Verification items for the finished model (mm, model axes). Face numbers are marked on the shaded views. Coordinates: 2 decimals unless noted, no trailing zeros. Write each loop counter-clockwise with the first axis right and the second up, starting at its lowest first coordinate (ties: lowest second). Pieces come first, ordered by that corner, then holes. Notation, with made-up numbers: (37.25, -5.5) - (50.25, -5.5) arc R9 ccw to (50.25, 8.5) - close; hole circle Ø4 at (-20.5, 58). An arc over 180 degrees is marked (long way). Use one line per item in the form item = value. Start each with the question number.
(1) Material ranges on line 1 (Z direction, x = 13.25, y = -5.5); line 2 (X direction, y = -7, z = 1.65); line 3 (X direction, y = -2, z = 0.5) (3 decimals), recorded low to high. Write a range as [from, to].
(2) Sectioned sample at C-C (x = 7.75). Record the cut outline in (y, z) (3 decimals), and give its area (3 significant figures).
(3) Sectioned sample at D-D (z = 3.75). Record the cut outline in (x, y), and give its area (3 significant figures).
(4) Gauge pin test, flat ends, axial feed: pin 1 Ø2.5 at (x, z) = (0, 2) entering from -Y; pin 2 Ø1.5 at (y, z) = (-5, 2.5) entering from -X; pin 3 Ø0.7 at (x, y) = (-0.5, -7) entering from +Z; pin 4 Ø0.6 at (x, y) = (3, -2) entering from -Z. Record the tip position at first contact, or that the pin passes through.
(5) Mould release check, pull along X, two halves, no side actions. Record for the marked faces 1, 2 and 3: released by +X, released by -X, zero draft, split by the parting line, or undercut.
(6) Sectioned sample at A-A (x = 0.5). Record the cut outline in (y, z).
(7) Sectioned sample at B-B (y = -3.25). Record the cut outline in (x, z) (3 decimals).
from build123d import *
from OCP.BRepFilletAPI import BRepFilletAPI_MakeChamfer

# Parameters (mm, degrees)
SKETCH_1_W             = 9.65
SKETCH_1_H             = 10.67
EXTRUDE_1_DEPTH        = 4.67
SKETCH_2_W             = 1.4
SKETCH_2_H             = 10.67
EXTRUDE_2_DEPTH        = 1.65
CHAMFER_1_SIZE         = 0.9
CHAMFER_1_SIZE2        = 2.472729678
CHAMFER_2_SIZE         = 3.22
CHAMFER_2_SIZE2        = 0.509997898
CHAMFER_3_SIZE         = 2.5
CHAMFER_3_SIZE2        = 0.395961101
FILLET_1_R             = 0.1
EXTRUDE_2_2_DEPTH      = 0.45
PATTERN_LINEAR_1_COUNT = 5
PATTERN_LINEAR_1_PITCH = 1.7


with BuildPart() as part:
    # Эскиз1 → Бобышка-Вытянуть1 (new body)
    with BuildSketch(Plane.XY):
        Rectangle(SKETCH_1_W, SKETCH_1_H)
    extrude(amount=EXTRUDE_1_DEPTH)

    # Эскиз2 → Extrude 2 (add)
    with BuildSketch(Plane(origin=(4.825, 0, 0), x_dir=(0, 0, -1), z_dir=(1, 0, 0))):
        with Locations((-0.7, 0)):
            Rectangle(SKETCH_2_W, SKETCH_2_H)
    extrude(amount=EXTRUDE_2_DEPTH)

    # Фаска1: one chamfer whose edges measure the first distance from different faces: ONE call of the kernel's chamfer builder (chamfer() names one face for all edges)
    chamfer_1_edges_1 = [part.edges().sort_by_distance(p)[0] for p in [
        (6.475, 5.335, 0.7),
    ]]
    chamfer_1_side_1 = [part.faces().sort_by_distance(p)[0] for p in [
        (0.275490496, 5.335, 2.255278414),
    ]]
    chamfer_1_edges_2 = [part.edges().sort_by_distance(p)[0] for p in [
        (6.475, -5.335, 0.7),
    ]]
    chamfer_1_side_2 = [part.faces().sort_by_distance(p)[0] for p in [
        (0.275490496, -5.335, 2.255278414),
    ]]
    chamfer_1 = BRepFilletAPI_MakeChamfer(part.part.solid().wrapped)
    for e in chamfer_1_edges_1:
        chamfer_1.Add(CHAMFER_1_SIZE, CHAMFER_1_SIZE2, e.wrapped, chamfer_1_side_1[0].wrapped)  # the first distance lies on this face
    for e in chamfer_1_edges_2:
        chamfer_1.Add(CHAMFER_1_SIZE, CHAMFER_1_SIZE2, e.wrapped, chamfer_1_side_2[0].wrapped)  # the first distance lies on this face
    add(Compound.cast(chamfer_1.Shape()), mode=Mode.REPLACE)

    # Фаска2: one chamfer whose edges measure the first distance from different faces: ONE call of the kernel's chamfer builder (chamfer() names one face for all edges)
    chamfer_2_edges_1 = [part.edges().sort_by_distance(p)[0] for p in [
        (0, -5.335, 4.67),
    ]]
    chamfer_2_side_1 = [part.faces().sort_by_distance(p)[0] for p in [
        (0.118398369, -5.335, 2.29777282),
    ]]
    chamfer_2_edges_2 = [part.edges().sort_by_distance(p)[0] for p in [
        (0, 5.335, 4.67),
    ]]
    chamfer_2_side_2 = [part.faces().sort_by_distance(p)[0] for p in [
        (0.118398369, 5.335, 2.29777282),
    ]]
    chamfer_2_edges_3 = [part.edges().sort_by_distance(p)[0] for p in [
        (4.825, 0, 4.67),
    ]]
    chamfer_2_side_3 = [part.faces().sort_by_distance(p)[0] for p in [
        (4.825, 0, 3.035),
    ]]
    chamfer_2 = BRepFilletAPI_MakeChamfer(part.part.solid().wrapped)
    for e in chamfer_2_edges_1:
        chamfer_2.Add(CHAMFER_2_SIZE, CHAMFER_2_SIZE2, e.wrapped, chamfer_2_side_1[0].wrapped)  # the first distance lies on this face
    for e in chamfer_2_edges_2:
        chamfer_2.Add(CHAMFER_2_SIZE, CHAMFER_2_SIZE2, e.wrapped, chamfer_2_side_2[0].wrapped)  # the first distance lies on this face
    for e in chamfer_2_edges_3:
        chamfer_2.Add(CHAMFER_2_SIZE, CHAMFER_2_SIZE2, e.wrapped, chamfer_2_side_3[0].wrapped)  # the first distance lies on this face
    add(Compound.cast(chamfer_2.Shape()), mode=Mode.REPLACE)

    # Фаска3
    chamfer_3_edges = [part.edges().sort_by_distance(p)[0] for p in [
        (-4.825, 0, 0),
    ]]
    chamfer_3_side = [part.faces().sort_by_distance(p)[0] for p in [
        (-4.825, 0, 2.292002655),
    ]]
    chamfer(chamfer_3_edges, length=CHAMFER_3_SIZE, length2=CHAMFER_3_SIZE2, reference=chamfer_3_side[0])

    # Скругление1
    fillet_1_edges = [part.edges().sort_by_distance(p)[0] for p in [
        (-4.825, 0, 4.67),
        (4.315002102, 0, 4.67),
        (-0.254998949, 4.825002102, 4.67),
        (-0.254998949, -4.825002102, 4.67),
    ]]
    fillet(fillet_1_edges, radius=FILLET_1_R)

    # Эскиз6 → Extrude 2 2 (add, symmetric)
    with BuildSketch(Plane(origin=(0, 3.4, 0), x_dir=(-1, 0, 0), z_dir=(0, 1, 0))):
        with BuildLine():
            Line((4.825, 2.47), (5.572169718, 2.47))
            ThreePointArc((5.572169718, 2.47), (6.020070605, 2.307944974), (6.26058695, 1.896813701))
            Line((6.26058695, 1.896813701), (6.50441305, 0.573186299))
            ThreePointArc((6.50441305, 0.573186299), (6.744929395, 0.162055026), (7.192830282, 0))
            Line((7.192830282, 0), (9.4, 0))
            Line((9.4, 0), (9.4, 0.58))
            Line((9.4, 0.58), (7.192830282, 0.58))
            ThreePointArc((7.192830282, 0.58), (7.116047273, 0.607780862), (7.074815899, 0.678260508))
            Line((7.074815899, 0.678260508), (6.830989799, 2.00188791))
            ThreePointArc((6.830989799, 2.00188791), (6.391188483, 2.75367081), (5.572169718, 3.05))
            Line((5.572169718, 3.05), (4.825, 3.05))
            Line((4.825, 3.05), (4.825, 2.47))
        make_face()
    extrude_2_2 = extrude(amount=EXTRUDE_2_2_DEPTH, both=True)

    # Линейный массив1: Extrude 2 2 ×5
    with Locations(*[(0, -i * PATTERN_LINEAR_1_PITCH, 0) for i in range(1, PATTERN_LINEAR_1_COUNT)]):
        add(extrude_2_2)


with BuildPart() as part_1:
    # Move Body 1: read off the stored shape, not the designer's step
    # Move Body 1: moved
    add(part.part.moved(Location((8.295, -3.4, 0))))


solid = part_1.part
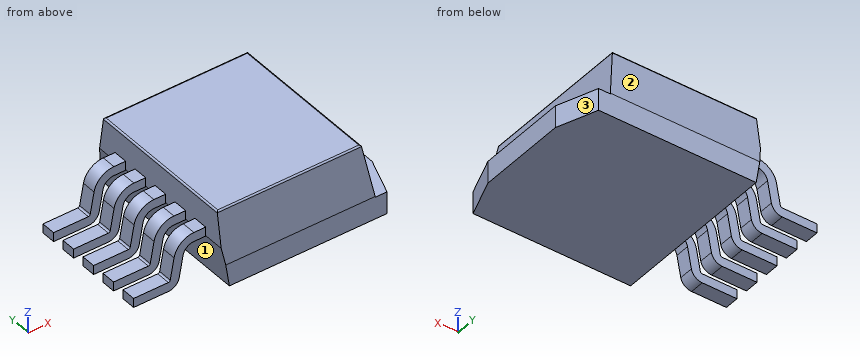
Answers below:
q1.line_1 = [0, 1.4]
q1.line_2 = [1.4, 1.99], [3.6, 13.09]
q1.line_3 = [-1.105, 1.773], [3.787, 14.77]
q2.outline = (-8.735, 0) - (1.935, 0) - (1.935, 1.45) - (1.438, 4.586) arc R0.1 ccw to (1.34, 4.67) - (-8.14, 4.67) arc R0.1 ccw to (-8.238, 4.586) - (-8.735, 1.45) - close
q2.area = 48.2 mm2
q3.outline = (3.47, -8.37) - (12.76, -8.37) - (12.76, 1.57) - (3.47, 1.57) - close
q3.area = 92.3 mm2
q4.pin_1 = through
q4.pin_2 = 1.42
q4.pin_3 = 0.58
q4.pin_4 = 2.47
q5.face_1 = undercut
q5.face_2 = zero draft
q5.face_3 = released by +X
q6.outline = (-7.25, 0) - (-6.35, 0) - (-6.35, 0.58) - (-7.25, 0.58) - close; (-5.55, 0) - (-4.65, 0) - (-4.65, 0.58) - (-5.55, 0.58) - close; (-3.85, 0) - (-2.95, 0) - (-2.95, 0.58) - (-3.85, 0.58) - close; (-2.15, 0) - (-1.25, 0) - (-1.25, 0.58) - (-2.15, 0.58) - close; (-0.45, 0) - (0.45, 0) - (0.45, 0.58) - (-0.45, 0.58) - close
q7.outline = (-1.105, 0) - (1.102, 0) arc R0.7 ccw to (1.791, 0.573) - (2.034, 1.897) arc R0.7 cw to (2.723, 2.47) - (3.47, 2.47) - (3.47, 2.5) - (3.866, 0) - (14.77, 0) - (14.77, 1.4) - (13.12, 1.4) - (13.12, 1.45) - (12.623, 4.586) arc R0.1 ccw to (12.525, 4.67) - (3.57, 4.67) arc R0.1 ccw to (3.47, 4.57) - (3.47, 3.05) - (2.723, 3.05) arc R1.28 ccw to (1.464, 2.002) - (1.22, 0.678) arc R0.12 cw to (1.102, 0.58) - (-1.105, 0.58) - close
